Read the model definition and answer for the solid it produces. Units are mm, in the model's axes. A direction names the side the tool comes from. Coordinates: 2 decimals unless noted, no trailing zeros. Order: outer loops, then holes, each group sorted by start corner. A loop starts at its lowest first (then second) coordinate and runs counter-clockwise, first axis right, second up. Notation, with made-up numbers: (49, 57) -> (89, 57) arc R25 ccw to (89, 78) -> close; hole circle Ø9 at (32, 23.25). An arc over 180 degrees is marked (long way). Use CSV: the item, a comma, the result in double quotes.
```python
from build123d import *

# Parameters (mm, degrees)
SKETCH060_W             = 50
SKETCH060_H             = 20
PAD059_DEPTH            = 5
SKETCH061_W             = 50
SKETCH061_H             = 3
PAD060_DEPTH            = 20
SKETCH062_W             = 50
SKETCH062_H             = 10
PAD061_DEPTH            = 3
BODY044_ROLL_ANGLE      = 150
BODY044_PLACEMENT_ANGLE = 180


with BuildPart() as part:
    # Sketch060 → Pad059 (new body)
    with BuildSketch(Plane.XY):
        with Locations((184.845276, -123.914059)):
            Rectangle(SKETCH060_W, SKETCH060_H)
    extrude(amount=PAD059_DEPTH)

    # Sketch061 (on Face6 of Pad059) → Pad060 (join)
    with BuildSketch(Plane.XY.offset(5)):
        with Locations((184.83606, -132.417099)):
            Rectangle(SKETCH061_W, SKETCH061_H)
    extrude(amount=PAD060_DEPTH)

    # Sketch062 (on Face7 of Pad060) → Pad061 (join)
    with BuildSketch(Plane(origin=(0, -113.914059, 0), x_dir=(-1, 0, 0), z_dir=(0, 1, 0))):
        with Locations((-184.841869, 9.989668)):
            Rectangle(SKETCH062_W, SKETCH062_H)
    extrude(amount=-PAD061_DEPTH)


with BuildPart() as part_1:
    # Body044 roll: moved
    add(part.part.rotate(Axis((0, 0, 0), (1, 0, 0)), BODY044_ROLL_ANGLE))


with BuildPart() as part_2:
    # Body044 placement: moved
    add(part_1.part.moved(Location((93.323153, 90.443186, 267.034204))).rotate(Axis((93.323153, 90.443186, 267.034204), (0, 0, 1)), BODY044_PLACEMENT_ANGLE))


solid = part_2.part
```
Item 1: Find section B-B, the plane z = 199.5. Give the vertices of the cut face in (x, y), then the cut area to 3 significant figures.
Return value:
outline,"(-116.52, -25.2) -> (-66.52, -25.2) -> (-66.52, -16.53) -> (-116.52, -16.53) -> close; (-116.52, -5.57) -> (-66.52, -5.57) -> (-66.52, -2.1) -> (-116.52, -2.1) -> close"
area,"607 mm^2"
Item 2: A tool of negligible diameter and unlimited length cuts with its end or side. For faces 4 (the flat face through (-91.172, -14.248, 200.817)), 5 (the flat face through (-91.172, -24.297, 197.942)), from which of +Z, -Z, +X, -X, +Y, -Y can it reach the whole face along a straight path? Write none if from no direction.
Return value:
face 4,"+X, -X"
face 5,"-Z, +X, -X, -Y"
Item 3: Straight lines are drawn through the part: line 1 along Y through (x, z) = (-104, 196); line 2 along Z through (x, y) = (-93, -14.5); line 3 along X through (y, z) = (-16.25, 188). For each, find the intervals that lie inside material, in ascending order.
Return value:
line 1,"y = -23.18 to -19.72, -3.55 to -2.61"
line 2,"z = 180.97 to 186.97, 200.67 to 206.45"
line 3,"x = -116.51 to -66.51"
Item 4: The mould has two halves that part along Y. Classify faces 1 (the flat face through (-91.87, -5.78, 199.87)), 2 (the flat face through (-91.163, -11.715, 179.186)), 3 (the flat face through (-116.519, -5, 201)): +Y half, -Y half, draft (parallel to the pull), parting line (faces both ways), or undercut.
Return value:
face 1,"undercut"
face 2,"+Y half"
face 3,"draft"
Item 5: Find section A-A, the plane y = -13.75. Give the vertices of the cut face in (x, z).
Return value:
outline,"(-116.52, 201.1) -> (-66.52, 201.1) -> (-66.52, 206.88) -> (-116.52, 206.88) -> close; (-116.51, 179.67) -> (-66.51, 179.67) -> (-66.51, 185.67) -> (-116.51, 185.67) -> close"
Item 6: Each of these flat-tipped pins is pushed along its axis until it touches: P1, Ø2, axis at x = -79.5, y = -16.5, coming from the +Z side; P2, Ø10, axis at x = -81.5, z = 192, coming from the +Y side; P3, Ø4, axis at x = -95.5, y = -13.5, coming from the +Z side; P4, Ø3, axis at y = -13, z = 199.5, coming from the +X side. Where does it stop, or does it pass through?
Return value:
P1,"stops at z = 205.87"
P2,"stops at y = -0.88"
P3,"stops at z = 208.18"
P4,"passes through"
